Work out the finished part from the listing and answer in its coordinate system (mm). A direction names the side the tool comes from. Round coordinates to 2 decimals unless told otherwise and drop trailing zeros. Order: outer loops, then holes, each group sorted by start corner. A loop starts at its lowest first (then second) coordinate and runs counter-clockwise, first axis right, second up. Notation, with made-up numbers: M -30,42.5 L -15,42.5 A24 ccw -15,70.5 Z; hole C 70,-26.5 d4. An arc over 180 degrees is marked long. Answer as a JSON object with one key per item and string values. Group by question number.
from build123d import *

# Parameters (mm, degrees)
ESBO_O1_R                = 7.5
ESBO_O1_R_2              = 4
RESSALTO_EXTRUS_O1_DEPTH = 12
ESBO_O2_R                = 7
ESBO_O2_R_2              = 4.5
CORTE_EXTRUS_O1_DEPTH    = 0.1
ESBO_O3_W                = 1.2
ESBO_O3_H                = 1


with BuildPart() as part:
    # Esboço1 → Ressalto-extrusão1 (new, symmetric)
    with BuildSketch(Plane.XY):
        Circle(ESBO_O1_R)
        Circle(ESBO_O1_R_2, mode=Mode.SUBTRACT)
    extrude(amount=RESSALTO_EXTRUS_O1_DEPTH, both=True)

    # Esboço2 → Corte-extrusão1 (cut)
    with BuildSketch(Plane.XY.offset(12)):
        Circle(ESBO_O2_R)
        Circle(ESBO_O2_R_2, mode=Mode.SUBTRACT)
    corte_extrus_o1 = extrude(amount=-CORTE_EXTRUS_O1_DEPTH, mode=Mode.SUBTRACT)

    # Espelhar1: Corte-extrusão1 across plane
    add(corte_extrus_o1.mirror(Plane.XY), mode=Mode.SUBTRACT)

    # Esboço3 → Corte-Revolução1 (revolve, cut)
    with BuildSketch(Plane(origin=(0, 0, 0), x_dir=(0, 0, -1), z_dir=(1, 0, 0)), mode=Mode.PRIVATE) as corte_revolu_o1_sk:
        with Locations((-8.1, 7.5)):
            Rectangle(ESBO_O3_W, ESBO_O3_H)
        with Locations((8.1, 7.5)):
            Rectangle(ESBO_O3_W, ESBO_O3_H)
    revolve(corte_revolu_o1_sk.sketch.rotate(Axis((0, 0, 0), (0, 0, 1)), 90), axis=Axis((0, 0, 0), (0, 0, 1)), mode=Mode.SUBTRACT)


solid = part.part
Item 1: Each of these flat-tipped pins is pushed along its axis until it touches: pin 1 (2 mm diameter, centred on y = -4, z = -6, fed in from -X); pin 2 (5 mm diameter, centred on y = 3.5, z = 1, fed in from -X); pin 3 (5 mm diameter, centred on x = -3.5, z = -3.5, fed in from -Y); pin 4 (6.5 mm diameter, centred on x = 0, y = 0, fed in from +Z). Where does it stop, or does it pass through?
Item 2: Find section B-B (y = 6.5). Give the vertices of the cut face in (x, z).
Item 3: Find section A-A (z = 10.5). Give the vertices of the cut face in (x, y), and give its area (3 significant figures).
Item 4: Consider L1, parallel to Y at x = 0, z = 11.95; L2, parallel to Y at x = 0, z = -3.5; L3, parallel to Y at x = 0, z = 8.25. Determine where each line is inside the solid, lowest interval first.
Item 5: The mould has two halves that part along Y. Classify faces 4 (the flat face through (-3, -3, 12)), 5 (the flat face through (0, -5, 11.9)), 6 (the cylindrical face through (-7.493, 0.33, -10.327)): +Y half, -Y half, draft (parallel to the pull), parting line (faces both ways), or undercut.
Item 6: A tool of negligible diameter and unlimited length cuts with its end or side. For faces 1 (the flat face through (0, -5, -11.9)), 2 (the flat face through (-3, -3, -12)), 3 (the flat face through (-2, 7, 7.5)), from which of +Z, -Z, +X, -X, +Y, -Y can it reach the whole face along a straight path? Write none if from no direction.
Responses:
{
 "1": {"pin 1": "stops at x = -6.87", "pin 2": "stops at x = -7.43", "pin 3": "stops at y = -7.43", "pin 4": "passes through"},
 "2": {"outline": "M -3.74,-12 L -2.6,-12 L -2.6,-11.9 L 2.6,-11.9 L 2.6,-12 L 3.74,-12 L 3.74,-8.7 L 2.6,-8.7 L 2.6,-7.5 L 3.74,-7.5 L 3.74,7.5 L 2.6,7.5 L 2.6,8.7 L 3.74,8.7 L 3.74,12 L 2.6,12 L 2.6,11.9 L -2.6,11.9 L -2.6,12 L -3.74,12 L -3.74,8.7 L -2.6,8.7 L -2.6,7.5 L -3.74,7.5 L -3.74,-7.5 L -2.6,-7.5 L -2.6,-8.7 L -3.74,-8.7 Z"},
 "3": {"outline": "C 0,0 d15; hole C 0,0 d8", "area": "126 mm^2"},
 "4": {"L1": "y = -7.5 to -7, -4.5 to -4, 4 to 4.5, 7 to 7.5", "L2": "y = -7.5 to -4, 4 to 7.5", "L3": "y = -7 to -4, 4 to 7"},
 "5": {"face 4": "draft", "face 5": "undercut", "face 6": "parting line"},
 "6": {"face 1": "-Z", "face 2": "-Z, +X, -X, +Y, -Y", "face 3": "none"}
}
